Autodesk Inventor part; units mm, degrees
ref_plane "YZ Plane" through (0, 0, 0) normal (1, 0, 0) x (0, 1, 0)
ref_plane "XZ Plane" through (0, 0, 0) normal (0, 1, 0) x (-1, 0, 0)
ref_plane "XY Plane" through (0, 0, 0) normal (0, 0, 1) x (1, 0, 0)
sketch "Sketch1" plane through (0, 0, 0) normal (0, 0, 1) x (1, 0, 0)
  line L0 (-25, 0) -> (25, 0)
  line L1 (25, 0) -> (83.737, 70)
  line L2 (83.737, 70) -> (99.0579, 57.1442)
  line L3 (99.0579, 57.1442) -> (34.3262, -20)
  line L4 (34.3262, -20) -> (-34.3262, -20)
  line L5 (-34.3262, -20) -> (-99.0579, 57.1442)
  line L6 (-99.0579, 57.1442) -> (-83.737, 70)
  line L7 (-83.737, 70) -> (-25, 0)
  line L8 (0, 0) -> (0, -20) construction
  dimension "d0" = 50
  dimension "d1" = 70
  dimension "d2" = 130
  dimension "d3" = 20
extrude "Plate1" add sketch "Sketch1" along normal blind 2
equation "\"d0\" = Лоток_ширина_низ"
equation "\"d1\" = Лоток_высота - Лоток_глубина_выреза"
equation "\"d2\" = Лоток_угол"
equation "\"d4\" = Thickness"
equation "\"BendRadius\" = Thickness"
equation "\"BendReliefWidth\" = Thickness"
equation "\"BendReliefDepth\" = 0.5 * Thickness"
equation "\"CornerReliefSize\" = 4 * Thickness"
equation "\"MinimumRemnant\" = 2 * Thickness"
equation "\"TransitionRadius\" = BendRadius"
equation "\"JacobiRadiusSize\" = BendRadius"
equation "\"GapSize\" = Thickness"
properties part number "ДМФ 044 фланец лотка"
The listing builds one solid part. Answer for the finished solid, in the listing's coordinates (mm). A direction names the side the tool comes from. Coordinates: 2 decimals unless noted, no trailing zeros. Loops run counter-clockwise (first coordinate to the right, second up) from the corner with the lowest first, then second, coordinate; pieces in that order, holes last. Notation, with made-up numbers: (70.5, 74.5) -> (119.5, 74.5) arc R23 ccw to (119.5, 96.5) -> close; hole circle Ø4 at (14, 27). An arc over 180 degrees is marked (long way). Use one line per item in the form item = value. Start each with the question number.
Item 1: The part is cut by section C-C on y = 39. Determine the outline of the cut face in (x, z), then the cut area to 3 significant figures.
Item 2: The part is cut by section A-A on y = 64. Determine the outline of the cut face in (x, z), then the cut area to 3 significant figures.
Item 3: The part is cut by section B-B on z = 0.65. Determine the outline of the cut face in (x, y), then the cut area to 3 significant figures.
Item 4: The mould has two halves that part along X. Classify faces 1 (the face through (53.957, 34.51, 0.986)), 2 (the face through (-66.239, 18.032, 0.986)), 3 (the face through (0, -1, 2)): released by +X, released by -X, zero draft, split by the parting line, or undercut.
Item 5: Consider L1, parallel to Y at x = -2, z = 1.7; L2, parallel to X at y = 36, z = 1.9; L3, parallel to X at y = 28, z = 0.2. Determine where each line is inside the solid, lowest interval first. Write a range as [from, to].
Item 6: A tool of negligible diameter and unlimited length cuts with its end or side. For faces 4 (the face through (-54.78, 35.49, 0.99)), 5 (the face through (-91.505, 63.482, 0.986)), from which of +Z, -Z, +X, -X, +Y, -Y can it reach the whole face along a straight path? Write none if from no direction.
Item 7: The part is cut by section D-D on x = -5.5. Determine the outline of the cut face in (y, z).
Answer key:
q1.outline = (-83.83, 0) -> (-57.72, 0) -> (-57.72, 2) -> (-83.83, 2) -> close; (57.72, 0) -> (83.83, 0) -> (83.83, 2) -> (57.72, 2) -> close
q1.area = 104 mm2
q2.outline = (-90.89, 0) -> (-78.7, 0) -> (-78.7, 2) -> (-90.89, 2) -> close; (78.7, 0) -> (90.89, 0) -> (90.89, 2) -> (78.7, 2) -> close
q2.area = 48.7 mm2
q3.outline = (-99.06, 57.14) -> (-34.33, -20) -> (34.33, -20) -> (99.06, 57.14) -> (83.74, 70) -> (25, 0) -> (-25, 0) -> (-83.74, 70) -> close
q3.area = 5,030 mm2
q4.face_1 = undercut
q4.face_2 = released by -X
q4.face_3 = zero draft
q5.L1 = [-20, 0]
q5.L2 = [-81.32, -55.21], [55.21, 81.32]
q5.L3 = [-74.6, -48.49], [48.49, 74.6]
q6.face_4 = +Z, -Z, +Y
q6.face_5 = +Z, -Z, -X, +Y
q7.outline = (-20, 0) -> (0, 0) -> (0, 2) -> (-20, 2) -> close
